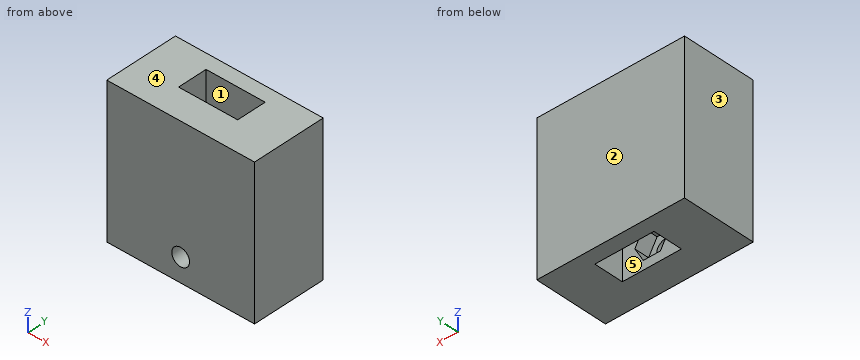
from build123d import *

# Parameters (mm, degrees)
SKETCH1_W           = 50
SKETCH1_H           = 50
BOSS_EXTRUDE1_DEPTH = 25
SKETCH2_W           = 20
SKETCH2_H           = 10
CUT_EXTRUDE1_DEPTH  = 50
SKETCH3_R           = 3
CUT_EXTRUDE2_DEPTH  = 10
CUT_EXTRUDE3_DEPTH  = 5


with BuildPart() as part:
    # Sketch1 → Boss-Extrude1 (new body)
    with BuildSketch(Plane(origin=(0, 0, 0), x_dir=(1, 0, 0), z_dir=(0, 1, 0))):
        with Locations((0, -25)):
            Rectangle(SKETCH1_W, SKETCH1_H)
    extrude(amount=BOSS_EXTRUDE1_DEPTH)

    # Sketch2 → Cut-Extrude1 (cut)
    with BuildSketch(Plane.XY.offset(50)):
        with Locations((0, 15)):
            Rectangle(SKETCH2_W, SKETCH2_H)
    extrude(amount=-CUT_EXTRUDE1_DEPTH, mode=Mode.SUBTRACT)

    # Sketch3 → Cut-Extrude2 (cut)
    with BuildSketch(Plane(origin=(0, 10, 0), x_dir=(1, 0, 0), z_dir=(0, 1, 0))):
        with Locations(Location((0, -8, 0), (0, 0, 270))):
            Circle(SKETCH3_R)
    extrude(amount=-CUT_EXTRUDE2_DEPTH, mode=Mode.SUBTRACT)

    # Sketch4 → Cut-Extrude3 (cut)
    with BuildSketch(Plane(origin=(0, 10, 0), x_dir=(1, 0, 0), z_dir=(0, 1, 0))):
        Polygon((2.886751346, -3), (-2.886751346, -3), (-5.773502692, -8), (-2.886751346, -13), (2.886751346, -13), (5.773502692, -8), align=None)
    extrude(amount=-CUT_EXTRUDE3_DEPTH, mode=Mode.SUBTRACT)


solid = part.part
Design review of the part built by this model. Coordinates are the model's own, in mm. Face numbers are marked on the shaded views. A direction names the side the tool comes from. Give positions to 0.01 mm unless a question says otherwise; leave off trailing zeros. Loops run counter-clockwise (first coordinate to the right, second up) from the corner with the lowest first, then second, coordinate; pieces in that order, holes last. Notation, with made-up numbers: M 72.5,56 L 91.5,56 A16 ccw 91.5,85 Z; hole C -37,-15 d6. An arc over 180 degrees is marked long. Write item = value, one per line.
Q1. To check wall thickness, follow line 1 (Y direction, x = 0, z = 29); line 2 (X direction, y = 13, z = 4.5); line 3 (X direction, y = 1.15, z = 8). State the ranges of each line that lie inside material, in increasing order. Write a range as [from, to].
Output values:
line_1 = [0, 10], [20, 25]
line_2 = [-25, -10], [10, 25]
line_3 = [-25, -3], [3, 25]
Q2. We need section A-A (x = 0). Give the boundary of the cut face in (y, z).
Output values:
outline = M 0,0 L 10,0 L 10,3 L 5,3 L 5,5 L 0,5 Z; M 0,11 L 5,11 L 5,13 L 10,13 L 10,50 L 0,50 Z; M 20,0 L 25,0 L 25,50 L 20,50 Z
Q3. Draft analysis for pull direction X (two halves, no side actions). For the marked faces 3, 4 and 5, state which applies: +X half, -X half, draft (parallel to the pull), parting line (faces both ways), or undercut.
Output values:
face_3 = -X half
face_4 = draft
face_5 = undercut
Q4. We need section D-D (y = 5.75). Give the boundary of the cut face in (x, z), plus the area to 3 significant figures.
Output values:
outline = M -25,0 L 25,0 L 25,50 L -25,50 Z; hole M -5.77,8 L -2.89,3 L 2.89,3 L 5.77,8 L 2.89,13 L -2.89,13 Z
area = 2,410 mm^2
Q5. For the marked faces 1 and 2, list the 3-axis set-ups (+Z, -Z, +X, -X, +Y, -Y) from which the entire face can be reached by the end or side of a thin tool; tool diameter is ignored.
Output values:
face_1 = +Z, -Z
face_2 = +Z, -Z, +X, -X, +Y
Q6. We need section B-B (z = 41.5). Give the boundary of the cut face in (x, y), plus the area to 3 significant figures.
Output values:
outline = M -25,0 L 25,0 L 25,25 L -25,25 Z; hole M -10,10 L 10,10 L 10,20 L -10,20 Z
area = 1,050 mm^2
Q7. We need section C-C (y = 14.75). Give the boundary of the cut face in (x, z).
Output values:
outline = M -25,0 L -10,0 L -10,50 L -25,50 Z; M 10,0 L 25,0 L 25,50 L 10,50 Z
